Verification items for the finished model (mm, model axes). A direction names the side the tool comes from. Give positions to 0.01 mm unless a question says otherwise; leave off trailing zeros. Order: outer loops, then holes, each group sorted by start corner. A loop starts at its lowest first (then second) coordinate and runs counter-clockwise, first axis right, second up.
(1) Sectioned sample at A-A on z = 0. Record the cut outline in (x, y), plus the area to 3 significant figures.
(2) Mould release check, pull along X, two halves, no side actions. Record for faces 1 (the face through (0, 986, 4.8)), 2 (the face through (0, 986, -4.4)): pulls with the +X half, pulls with the -X half, needs draft (parallel to the pull), parting line crosses it, or undercut.
(3) Gauge pin test, flat ends, axial feed: pin 1 (4 mm diameter, centred on y = 1146, z = 3.5, fed in from +X); pin 2 (2 mm diameter, centred on y = 979, z = -2, fed in from -X). Record the tip position at first contact, or that the pin passes through.
(4) Scan lines: L1, parallel to Z at x = -8, y = 337.5; L2, parallel to X at y = 590, z = 1.5; L3, parallel to X at y = 566, z = 1.25. Record each from-to range of solid material in increasing order.
(5) Sectioned sample at B-B on y = 192.5. Record the cut outline in (x, z).
(6) Sectioned sample at C-C on x = -9.5. Record the cut outline in (y, z).
(7) Access from +Z, -Z, +X, -X, +Y, -Y to the whole of each face (thin tool, end or side, straight path). Record for faces 3 (the face through (0, 986, -4.8)), 4 (the face through (0, 986, 4.4)).
Autodesk Inventor part; units mm, degrees
ref_plane "YZ Plane" through (0, 0, 0) normal (1, 0, 0) x (0, 1, 0)
ref_plane "XZ Plane" through (0, 0, 0) normal (0, 1, 0) x (-1, 0, 0)
ref_plane "XY Plane" through (0, 0, 0) normal (0, 0, 1) x (1, 0, 0)
sketch "Эскиз1" plane through (0, 0, 0) normal (0, 1, 0) x (-1, 0, 0)
  line L0 (18.7, 4.8) -> (-18.7, 4.8)
  line L1 (-23.5, 0) -> (-23.5, 0)
  line L2 (-18.7, -4.8) -> (18.7, -4.8)
  line L3 (23.5, 0) -> (23.5, 0)
  arc A0 (23.5, 0) -> (18.7, 4.8) centre (18.7, 0) ccw
  arc A1 (18.7, -4.8) -> (23.5, 0) centre (18.7, 0) ccw
  arc A2 (-18.7, 4.8) -> (-23.5, 0) centre (-18.7, 0) ccw
  arc A3 (-23.5, 0) -> (-18.7, -4.8) centre (-18.7, 0) ccw
  line L4 (18.7, 4.4) -> (-18.7, 4.4)
  line L5 (-23.1, 0) -> (-23.1, 0)
  line L6 (-18.7, -4.4) -> (18.7, -4.4)
  line L7 (23.1, 0) -> (23.1, 0)
  arc A4 (23.1, 0) -> (18.7, 4.4) centre (18.7, 0) ccw
  arc A5 (18.7, -4.4) -> (23.1, 0) centre (18.7, 0) ccw
  arc A6 (-23.1, 0) -> (-18.7, -4.4) centre (-18.7, 0) ccw
  arc A7 (-18.7, 4.4) -> (-23.1, 0) centre (-18.7, 0) ccw
  point P0 (0, 0)
  dimension "d0" = 4.8
  dimension "d1" = 4.8
  dimension "d2" = 47
  dimension "d3" = 23.5
  dimension "d4" = 4.8
  dimension "d5" = 4.4
  dimension "d6" = 4.4
  dimension "d7" = 23.1
  dimension "d8" = 23.1
  dimension "d9" = 4.4
extrude "Выдавливание1" add sketch "Эскиз1" along normal blind 2000
properties part number "isolation"
Ans:
1. outline: (-23.5, 0) - (-23.1, 0) - (-23.1, 2000) - (-23.5, 2000) - close; (23.1, 0) - (23.5, 0) - (23.5, 2000) - (23.1, 2000) - close
1. area: 1,600 mm2
2. face 1: needs draft
2. face 2: undercut
3. pin 1: stops at x = 23.26
3. pin 2: stops at x = -23.39
4. L1: z = -4.8 to -4.4, 4.4 to 4.8
4. L2: x = -23.26 to -22.84, 22.84 to 23.26
4. L3: x = -23.33 to -22.92, 22.92 to 23.33
5. outline: (-18.7, -4.8) - (18.7, -4.8) arc R4.8 ccw to (18.7, 4.8) - (-18.7, 4.8) arc R4.8 ccw to start; hole (-18.7, -4.4) - (18.7, -4.4) arc R4.4 ccw to (18.7, 4.4) - (-18.7, 4.4) arc R4.4 ccw to start
6. outline: (0, -4.8) - (2000, -4.8) - (2000, -4.4) - (0, -4.4) - close; (0, 4.4) - (2000, 4.4) - (2000, 4.8) - (0, 4.8) - close
7. face 3: -Z, +X, -X, +Y, -Y
7. face 4: +Y, -Y
